Part print with two shaded views. Sizes in mm from the minimum x, y, z corner. A direction names the side the tool comes from. Coordinates: 2 decimals unless noted, no trailing zeros. Order: outer loops, then holes, each group sorted by start corner. A loop starts at its lowest first (then second) coordinate and runs counter-clockwise, first axis right, second up. Notation, with made-up numbers: (-18, 2) - (3, 2) arc R15 cw to (3, 8) - close; hole circle Ø6 at (-5, 35). An arc over 180 degrees is marked (long way). Return JSON: item names as keys, results as strings.
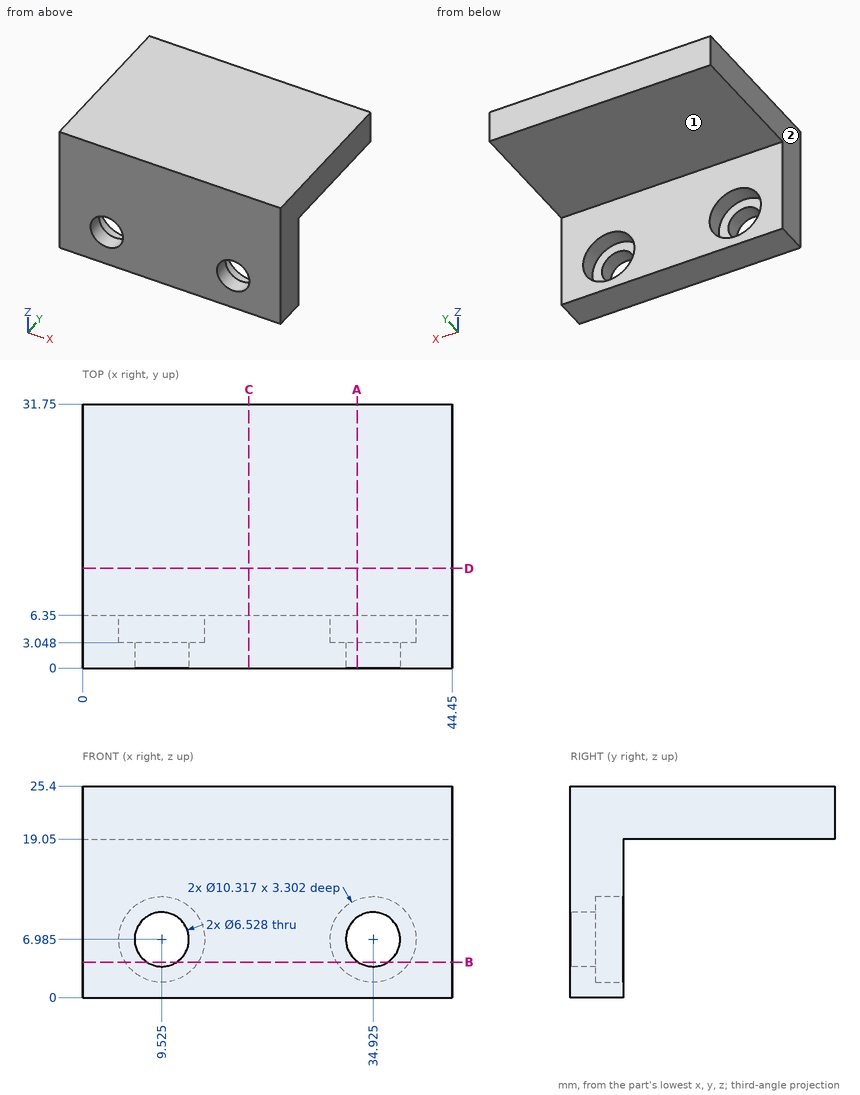
Item 1: Band-saw the part on B-B, the plane z = 4.25. List the corners of the cut face in (x, y).
Findings below:
{"outline": "(0, 0) - (7.74, 0) - (7.74, 3.05) - (5.15, 3.05) - (5.15, 6.35) - (0, 6.35) - close; (11.31, 0) - (33.14, 0) - (33.14, 3.05) - (30.55, 3.05) - (30.55, 6.35) - (13.9, 6.35) - (13.9, 3.05) - (11.31, 3.05) - close; (36.71, 0) - (44.45, 0) - (44.45, 6.35) - (39.3, 6.35) - (39.3, 3.05) - (36.71, 3.05) - close"}
Item 2: Band-saw the part on D-D, the plane y = 12. List the corners of the cut face in (x, z).
Findings below:
{"outline": "(0, 19.05) - (44.45, 19.05) - (44.45, 25.4) - (0, 25.4) - close"}
Item 3: Drop flat-ended pins along their axis: P1, Ø8, axis at x = 15, y = 13.5, coming from the -Z side; P2, Ø1, axis at x = 27.5, y = 4.5, coming from the -Z side; P3, Ø8.5, axis at x = 34.5, z = 5, coming from the +Y side. Give the stop position or say it passes through.
Findings below:
{"P1": "stops at z = 19.05", "P2": "stops at z = 0", "P3": "stops at y = 6.35"}
Item 4: Band-saw the part on A-A, the plane x = 33. List the corners of the cut face in (y, z).
Findings below:
{"outline": "(0, 0) - (6.35, 0) - (6.35, 2.2) - (3.05, 2.2) - (3.05, 4.35) - (0, 4.35) - close; (0, 9.62) - (3.05, 9.62) - (3.05, 11.77) - (6.35, 11.77) - (6.35, 19.05) - (31.75, 19.05) - (31.75, 25.4) - (0, 25.4) - close"}
Item 5: Wall check: L1, parallel to Y at x = 3, z = 9.5; L2, parallel to Z at x = 20, y = 18; L3, parallel to X at y = 4.5, z = 9.25. Give the ranges that are in metal, low to high. Write a range as [from, to].
Findings below:
{"L1": "y = [0, 6.35]", "L2": "z = [19.05, 25.4]", "L3": "x = [0, 4.89], [14.16, 30.29], [39.56, 44.45]"}
Item 6: Which spindle directions (+Z, -Z, +X, -X, +Y, -Y) get a long thin tool onto all of the face, cutting with end or side? Do the marked faces 1 and 2. Say none if no direction does.
Findings below:
{"face 1": "-Z, +X, -X, +Y", "face 2": "+Z, -Z, -X, +Y, -Y"}
Item 7: Band-saw the part on C-C, the plane x = 20. List the corners of the cut face in (y, z).
Findings below:
{"outline": "(0, 0) - (6.35, 0) - (6.35, 19.05) - (31.75, 19.05) - (31.75, 25.4) - (0, 25.4) - close"}
